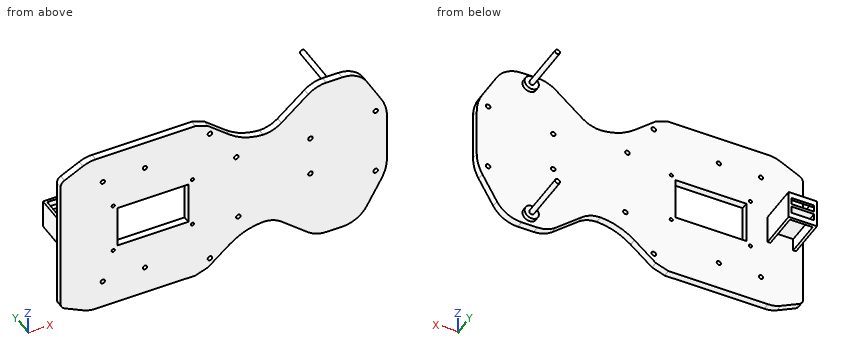
```python
from build123d import *
from OCP.BRepFilletAPI import BRepFilletAPI_MakeChamfer

# Parameters (mm, degrees)
BOSS_EXTRUDE1_DEPTH = 5
CHAMFER1_SIZE       = 5
CHAMFER1_SIZE2      = 5.047084744
FILLET4_R           = 20
FILLET5_R           = 30
FILLET6_R           = 20
FILLET7_R           = 40
FILLET8_R           = 20
FILLET9_R           = 5
CUT_EXTRUDE3_REACH  = 154.398
SKETCH7_R           = 1.5
SKETCH3_R           = 1.75
BOSS_EXTRUDE2_DEPTH = 37.5
SKETCH8_R           = 5
BOSS_EXTRUDE3_DEPTH = 3
SKETCH9_W           = 20
SKETCH9_H           = 20
BOSS_EXTRUDE4_DEPTH = 28
SKETCH12_W          = 16
SKETCH12_H          = 5
CUT_EXTRUDE5_DEPTH  = 28
CUT_EXTRUDE7_REACH  = 164.192
SKETCH13_W          = 16
SKETCH13_H          = 26
CUT_EXTRUDE8_REACH  = 158.864
SKETCH15_R          = 1.125
CUT_EXTRUDE10_REACH = 158.864
SKETCH16_W          = 50
SKETCH16_H          = 30
CUT_EXTRUDE11_REACH = 158.864
SKETCH17_R          = 1.6
CUT_EXTRUDE12_REACH = 158.864
SKETCH18_R          = 1.6
CUT_EXTRUDE13_REACH = 158.864
SKETCH19_R          = 1.6


with BuildPart() as part:
    # Sketch1 → Boss-Extrude1 (new body)
    with BuildSketch(Plane(origin=(0, 0, 0), x_dir=(1, 0, 0), z_dir=(0, 1, 0))):
        Polygon((40, 60), (70, 60), (90, 25), (90, -25), (70, -60), (40, -60), (10, -35), (-10, -35), (-40, -60), (-120, -60), (-140, -50), (-140, 50), (-120, 60), (-40, 60), (-10, 35), (10, 35), align=None)
    extrude(amount=BOSS_EXTRUDE1_DEPTH)

    # Chamfer1: one chamfer whose edges measure the first distance from different faces: ONE call of the kernel's chamfer builder (chamfer() names one face for all edges)
    chamfer1_edges_1 = [part.edges().sort_by_distance(p)[0] for p in [
        (-40, 2.5, 60),
    ]]
    chamfer1_side_1 = [part.faces().sort_by_distance(p)[0] for p in [
        (-80, 2.5, 60),
    ]]
    chamfer1_edges_2 = [part.edges().sort_by_distance(p)[0] for p in [
        (-40, 2.5, -60),
    ]]
    chamfer1_side_2 = [part.faces().sort_by_distance(p)[0] for p in [
        (-25, 2.5, -47.5),
    ]]
    chamfer1 = BRepFilletAPI_MakeChamfer(part.part.solid().wrapped)
    for e in chamfer1_edges_1:
        chamfer1.Add(CHAMFER1_SIZE, CHAMFER1_SIZE2, e.wrapped, chamfer1_side_1[0].wrapped)  # the first distance lies on this face
    for e in chamfer1_edges_2:
        chamfer1.Add(CHAMFER1_SIZE, CHAMFER1_SIZE2, e.wrapped, chamfer1_side_2[0].wrapped)  # the first distance lies on this face
    add(Compound.cast(chamfer1.Shape()), mode=Mode.REPLACE)

    # Fillet4
    fillet4_edges = [part.edges().sort_by_distance(p)[0] for p in [
        (40, 2.5, -60),
        (70, 2.5, -60),
        (70, 2.5, 60),
        (40, 2.5, 60),
    ]]
    fillet(fillet4_edges, radius=FILLET4_R)

    # Fillet5
    fillet5_edges = [part.edges().sort_by_distance(p)[0] for p in [
        (90, 2.5, -25),
        (90, 2.5, 25),
    ]]
    fillet(fillet5_edges, radius=FILLET5_R)

    # Fillet6
    fillet6_edges = [part.edges().sort_by_distance(p)[0] for p in [
        (10, 2.5, 35),
        (10, 2.5, -35),
    ]]
    fillet(fillet6_edges, radius=FILLET6_R)

    # Fillet7
    # the kernel refuses this fillet: 40 mm, written as the material it adds along each edge
    with BuildSketch(Plane(origin=(-10, 0, -35), x_dir=(-0.768221279597376, 0, -0.6401843996644798), z_dir=(0, 1, 0))) as fillet7_piece_1:
        with BuildLine():
            CenterArc((14.420794682, -40), FILLET7_R, 90, 37.26938559)
            Line((-9.801736302, -8.168113585), (0, 0))
            Line((0, 0), (14.420794682, 0))
        make_face()
    extrude(amount=5)
    with BuildSketch(Plane(origin=(-10, 0, 35), x_dir=(1, 0, 0), z_dir=(0, 1, 0))) as fillet7_piece_2:
        with BuildLine():
            CenterArc((14.529014643, -39.96081897), FILLET7_R, 92.536185502, 37.26938559)
            Line((-11.078361343, -9.231967786), (0, 0))
            Line((0, 0), (12.759001296, 0))
        make_face()
    extrude(amount=5)

    # Fillet8
    fillet8_edges = [part.edges().sort_by_distance(p)[0] for p in [
        (-120, 2.5, 60),
        (-120, 2.5, -60),
    ]]
    fillet(fillet8_edges, radius=FILLET8_R)

    # Fillet9
    fillet9_edges = [part.edges().sort_by_distance(p)[0] for p in [
        (-140, 2.5, 50),
        (-140, 2.5, -50),
    ]]
    fillet(fillet9_edges, radius=FILLET9_R)

    # Sketch7 → Cut-Extrude3 (cut, up to next)
    with BuildSketch(Plane(origin=(0, 5, 0), x_dir=(1, 0, 0), z_dir=(0, 1, 0)), mode=Mode.PRIVATE) as cut_extrude3_sk1:
        with Locations(Location((-110.27864045, 40, 0), (0, 0, 270))):
            Circle(SKETCH7_R)
    cut_extrude3_tool1 = extrude(cut_extrude3_sk1.sketch, amount=-CUT_EXTRUDE3_REACH, mode=Mode.PRIVATE) & part.part
    # Sketch7 → Cut-Extrude3 (cut, up to next)
    with BuildSketch(Plane(origin=(0, 5, 0), x_dir=(1, 0, 0), z_dir=(0, 1, 0)), mode=Mode.PRIVATE) as cut_extrude3_sk2:
        with Locations(Location((-80.57864045, 40, 0), (0, 0, 270))):
            Circle(SKETCH7_R)
    cut_extrude3_tool2 = extrude(cut_extrude3_sk2.sketch, amount=-CUT_EXTRUDE3_REACH, mode=Mode.PRIVATE) & part.part
    cut_extrude3_1 = cut_extrude3_tool1.solids().sort_by_distance((-110.27864, 5, -40))[0]
    add(cut_extrude3_1, mode=Mode.SUBTRACT)
    cut_extrude3_2 = cut_extrude3_tool2.solids().sort_by_distance((-80.57864, 5, -40))[0]
    add(cut_extrude3_2, mode=Mode.SUBTRACT)
    cut_extrude3 = cut_extrude3_1 + cut_extrude3_2  # Cut-Extrude3 as one shape, for the pattern or mirror that repeats it

    # Mirror1: Cut-Extrude3 across plane
    add(cut_extrude3.mirror(Plane.XY), mode=Mode.SUBTRACT)

    # Sketch3 → Boss-Extrude2 (add)
    with BuildSketch(Plane(origin=(0, 5, 0), x_dir=(1, 0, 0), z_dir=(0, 1, 0))):
        with Locations(Location((52.817273997, 52, 0), (0, 0, 270))):
            Circle(SKETCH3_R)
        with Locations(Location((52.817273997, -52, 0), (0, 0, 270))):
            Circle(SKETCH3_R)
    extrude(amount=BOSS_EXTRUDE2_DEPTH)

    # Sketch8 → Boss-Extrude3 (add)
    with BuildSketch(Plane(origin=(0, 5, 0), x_dir=(1, 0, 0), z_dir=(0, 1, 0))):
        with Locations(Location((52.817273997, 52, 0), (0, 0, 270))):
            Circle(SKETCH8_R)
        with Locations(Location((52.817273997, -52, 0), (0, 0, 270))):
            Circle(SKETCH8_R)
    extrude(amount=BOSS_EXTRUDE3_DEPTH)

    # Sketch9 → Boss-Extrude4 (add)
    with BuildSketch(Plane(origin=(0, 5, 0), x_dir=(1, 0, 0), z_dir=(0, 1, 0))):
        with Locations((-125, 0)):
            Rectangle(SKETCH9_W, SKETCH9_H)
    extrude(amount=BOSS_EXTRUDE4_DEPTH)

    # Sketch12 → Cut-Extrude5 (cut)
    with BuildSketch(Plane(origin=(0, 33, 0), x_dir=(1, 0, 0), z_dir=(0, 1, 0))):
        with Locations((-125, -3.5)):
            Rectangle(SKETCH12_W, SKETCH12_H)
        with Locations((-125, 3.5)):
            Rectangle(SKETCH12_W, SKETCH12_H)
    extrude(amount=-CUT_EXTRUDE5_DEPTH, mode=Mode.SUBTRACT)

    # Sketch13 → Cut-Extrude7 (cut, up to next)
    with BuildSketch(Plane(origin=(0, 0, -10), x_dir=(-1, 0, 0), z_dir=(0, 0, -1)), mode=Mode.PRIVATE) as cut_extrude7_sk1:
        with Locations((125, 18)):
            Rectangle(SKETCH13_W, SKETCH13_H)
    cut_extrude7_tool1 = extrude(cut_extrude7_sk1.sketch, amount=-CUT_EXTRUDE7_REACH, mode=Mode.PRIVATE) & part.part
    cut_extrude7 = cut_extrude7_tool1.solids().sort_by_distance((-125, 18, -10))[0]
    add(cut_extrude7, mode=Mode.SUBTRACT)

    # Mirror2: Cut-Extrude7 across plane
    add(cut_extrude7.mirror(Plane.XY), mode=Mode.SUBTRACT)

    # Sketch15 → Cut-Extrude8 (cut, up to next)
    with BuildSketch(Plane(origin=(0, 5, 0), x_dir=(1, 0, 0), z_dir=(0, 1, 0)), mode=Mode.PRIVATE) as cut_extrude8_sk1:
        with Locations(Location((-102.875, 17.875, 0), (0, 0, 270))):
            Circle(SKETCH15_R)
    cut_extrude8_tool1 = extrude(cut_extrude8_sk1.sketch, amount=-CUT_EXTRUDE8_REACH, mode=Mode.PRIVATE) & part.part
    # Sketch15 → Cut-Extrude8 (cut, up to next)
    with BuildSketch(Plane(origin=(0, 5, 0), x_dir=(1, 0, 0), z_dir=(0, 1, 0)), mode=Mode.PRIVATE) as cut_extrude8_sk2:
        with Locations(Location((-102.875, -17.875, 0), (0, 0, 270))):
            Circle(SKETCH15_R)
    cut_extrude8_tool2 = extrude(cut_extrude8_sk2.sketch, amount=-CUT_EXTRUDE8_REACH, mode=Mode.PRIVATE) & part.part
    # Sketch15 → Cut-Extrude8 (cut, up to next)
    with BuildSketch(Plane(origin=(0, 5, 0), x_dir=(1, 0, 0), z_dir=(0, 1, 0)), mode=Mode.PRIVATE) as cut_extrude8_sk3:
        with Locations(Location((-47.125, -17.875, 0), (0, 0, 270))):
            Circle(SKETCH15_R)
    cut_extrude8_tool3 = extrude(cut_extrude8_sk3.sketch, amount=-CUT_EXTRUDE8_REACH, mode=Mode.PRIVATE) & part.part
    # Sketch15 → Cut-Extrude8 (cut, up to next)
    with BuildSketch(Plane(origin=(0, 5, 0), x_dir=(1, 0, 0), z_dir=(0, 1, 0)), mode=Mode.PRIVATE) as cut_extrude8_sk4:
        with Locations(Location((-47.125, 17.875, 0), (0, 0, 270))):
            Circle(SKETCH15_R)
    cut_extrude8_tool4 = extrude(cut_extrude8_sk4.sketch, amount=-CUT_EXTRUDE8_REACH, mode=Mode.PRIVATE) & part.part
    add(cut_extrude8_tool1.solids().sort_by_distance((-102.875, 5, -17.875))[0], mode=Mode.SUBTRACT)
    add(cut_extrude8_tool2.solids().sort_by_distance((-102.875, 5, 17.875))[0], mode=Mode.SUBTRACT)
    add(cut_extrude8_tool3.solids().sort_by_distance((-47.125, 5, 17.875))[0], mode=Mode.SUBTRACT)
    add(cut_extrude8_tool4.solids().sort_by_distance((-47.125, 5, -17.875))[0], mode=Mode.SUBTRACT)

    # Sketch16 → Cut-Extrude10 (cut, up to next)
    with BuildSketch(Plane(origin=(0, 5, 0), x_dir=(1, 0, 0), z_dir=(0, 1, 0)), mode=Mode.PRIVATE) as cut_extrude10_sk1:
        with Locations((-75, 0)):
            Rectangle(SKETCH16_W, SKETCH16_H)
    cut_extrude10_tool1 = extrude(cut_extrude10_sk1.sketch, amount=-CUT_EXTRUDE10_REACH, mode=Mode.PRIVATE) & part.part
    add(cut_extrude10_tool1.solids().sort_by_distance((-75, 5, 0))[0], mode=Mode.SUBTRACT)

    # Sketch17 → Cut-Extrude11 (cut, up to next)
    with BuildSketch(Plane(origin=(0, 5, 0), x_dir=(1, 0, 0), z_dir=(0, 1, 0)), mode=Mode.PRIVATE) as cut_extrude11_sk1:
        with Locations(Location((-14.75, 24.16, 0), (0, 0, 270))):
            Circle(SKETCH17_R)
    cut_extrude11_tool1 = extrude(cut_extrude11_sk1.sketch, amount=-CUT_EXTRUDE11_REACH, mode=Mode.PRIVATE) & part.part
    # Sketch17 → Cut-Extrude11 (cut, up to next)
    with BuildSketch(Plane(origin=(0, 5, 0), x_dir=(1, 0, 0), z_dir=(0, 1, 0)), mode=Mode.PRIVATE) as cut_extrude11_sk2:
        with Locations(Location((-16.2, -24.15, 0), (0, 0, 270))):
            Circle(SKETCH17_R)
    cut_extrude11_tool2 = extrude(cut_extrude11_sk2.sketch, amount=-CUT_EXTRUDE11_REACH, mode=Mode.PRIVATE) & part.part
    # Sketch17 → Cut-Extrude11 (cut, up to next)
    with BuildSketch(Plane(origin=(0, 5, 0), x_dir=(1, 0, 0), z_dir=(0, 1, 0)), mode=Mode.PRIVATE) as cut_extrude11_sk3:
        with Locations(Location((36.06, -19.34, 0), (0, 0, 270))):
            Circle(SKETCH17_R)
    cut_extrude11_tool3 = extrude(cut_extrude11_sk3.sketch, amount=-CUT_EXTRUDE11_REACH, mode=Mode.PRIVATE) & part.part
    # Sketch17 → Cut-Extrude11 (cut, up to next)
    with BuildSketch(Plane(origin=(0, 5, 0), x_dir=(1, 0, 0), z_dir=(0, 1, 0)), mode=Mode.PRIVATE) as cut_extrude11_sk4:
        with Locations(Location((36.06, 8.83, 0), (0, 0, 270))):
            Circle(SKETCH17_R)
    cut_extrude11_tool4 = extrude(cut_extrude11_sk4.sketch, amount=-CUT_EXTRUDE11_REACH, mode=Mode.PRIVATE) & part.part
    add(cut_extrude11_tool1.solids().sort_by_distance((-14.75, 5, -24.16))[0], mode=Mode.SUBTRACT)
    add(cut_extrude11_tool2.solids().sort_by_distance((-16.2, 5, 24.15))[0], mode=Mode.SUBTRACT)
    add(cut_extrude11_tool3.solids().sort_by_distance((36.06, 5, 19.34))[0], mode=Mode.SUBTRACT)
    add(cut_extrude11_tool4.solids().sort_by_distance((36.06, 5, -8.83))[0], mode=Mode.SUBTRACT)

    # Sketch18 → Cut-Extrude12 (cut, up to next)
    with BuildSketch(Plane(origin=(0, 5, 0), x_dir=(1, 0, 0), z_dir=(0, 1, 0)), mode=Mode.PRIVATE) as cut_extrude12_sk1:
        with Locations(Location((82, 24, 0), (0, 0, 270))):
            Circle(SKETCH18_R)
    cut_extrude12_tool1 = extrude(cut_extrude12_sk1.sketch, amount=-CUT_EXTRUDE12_REACH, mode=Mode.PRIVATE) & part.part
    # Sketch18 → Cut-Extrude12 (cut, up to next)
    with BuildSketch(Plane(origin=(0, 5, 0), x_dir=(1, 0, 0), z_dir=(0, 1, 0)), mode=Mode.PRIVATE) as cut_extrude12_sk2:
        with Locations(Location((82, -24, 0), (0, 0, 270))):
            Circle(SKETCH18_R)
    cut_extrude12_tool2 = extrude(cut_extrude12_sk2.sketch, amount=-CUT_EXTRUDE12_REACH, mode=Mode.PRIVATE) & part.part
    add(cut_extrude12_tool1.solids().sort_by_distance((82, 5, -24))[0], mode=Mode.SUBTRACT)
    add(cut_extrude12_tool2.solids().sort_by_distance((82, 5, 24))[0], mode=Mode.SUBTRACT)

    # Sketch19 → Cut-Extrude13 (cut, up to next)
    with BuildSketch(Plane(origin=(0, 5, 0), x_dir=(1, 0, 0), z_dir=(0, 1, 0)), mode=Mode.PRIVATE) as cut_extrude13_sk1:
        with Locations(Location((-34.75, -50, 0), (0, 0, 270))):
            Circle(SKETCH19_R)
    cut_extrude13_tool1 = extrude(cut_extrude13_sk1.sketch, amount=-CUT_EXTRUDE13_REACH, mode=Mode.PRIVATE) & part.part
    # Sketch19 → Cut-Extrude13 (cut, up to next)
    with BuildSketch(Plane(origin=(0, 5, 0), x_dir=(1, 0, 0), z_dir=(0, 1, 0)), mode=Mode.PRIVATE) as cut_extrude13_sk2:
        with Locations(Location((-34.75, 50, 0), (0, 0, 270))):
            Circle(SKETCH19_R)
    cut_extrude13_tool2 = extrude(cut_extrude13_sk2.sketch, amount=-CUT_EXTRUDE13_REACH, mode=Mode.PRIVATE) & part.part
    add(cut_extrude13_tool1.solids().sort_by_distance((-34.75, 5, 50))[0], mode=Mode.SUBTRACT)
    add(cut_extrude13_tool2.solids().sort_by_distance((-34.75, 5, -50))[0], mode=Mode.SUBTRACT)


solid = part.part
```
Geometry check sheet. Reference: the model listing, model coordinates, mm. Coordinates: 2 decimals unless noted, no trailing zeros. Loops run counter-clockwise (first coordinate to the right, second up) from the corner with the lowest first, then second, coordinate; pieces in that order, holes last. Notation, with made-up numbers: (13.5, 35.5) - (30.5, 35.5) arc R10 cw to (30.5, 51.5) - close; hole circle Ø1 at (25.5, 65). An arc over 180 degrees is marked (long way). One line per item, written item: value. Start each with the question number.
(1) Material ranges on line 1 (X direction, y = 2.7, z = 24.15); line 2 (X direction, y = 1, z = -24); line 3 (Z direction, x = 82, y = 3.45), recorded low to high. Write a range as [from, to].
(2) Cross-section at C-C on x = 9. Enter the section's corners in (y, z).
(3) Cross-section at B-B on y = 26.5. Enter the section's corners in (x, z), plus the area to 3 significant figures.
(4) Depth check by flat-ended pin: P1, Ø2.5, axis at y = 21.5, z = -4.5, coming from the -X side; P2, Ø22, axis at x = -120.5, y = 21.5, coming from the -Z side; P3, Ø5, axis at x = 36.06, z = -8.83, coming from the +Y side; P4, Ø1.9, axis at x = 82, z = 24, coming from the -Y side. Enter the tip coordinate at first touch or a pass-through.
(5) Cross-section at A-A on x = -71. Enter the section's corners in (y, z).
Results below:
1. line 1: x = [-140, -17.8], [-14.6, 80.41], [83.59, 89.14]
1. line 2: x = [-140, -16.34], [-13.16, 80.4], [83.6, 89.18]
1. line 3: z = [-39, -25.6], [-22.4, 22.4], [25.6, 39]
2. outline: (0, -36) - (5, -36) - (5, 36) - (0, 36) - close
3. outline: (-135, -10) - (-133, -10) - (-133, -1) - (-117, -1) - (-117, -10) - (-115, -10) - (-115, 10) - (-117, 10) - (-117, 1) - (-133, 1) - (-133, 10) - (-135, 10) - close; circle Ø3.5 at (52.82, -52); circle Ø3.5 at (52.82, 52)
3. area: 131 mm2
4. P1: stops at x = -135
4. P2: stops at z = -10
4. P3: stops at y = 5
4. P4: passes through
5. outline: (0, -60) - (5, -60) - (5, -15) - (0, -15) - close; (0, 15) - (5, 15) - (5, 60) - (0, 60) - close
